Geometry check sheet. Reference: the model listing, model coordinates, mm. Face numbers are marked on the shaded views. A direction names the side the tool comes from. Round coordinates to 2 decimals unless told otherwise and drop trailing zeros. Order: outer loops, then holes, each group sorted by start corner. A loop starts at its lowest first (then second) coordinate and runs counter-clockwise, first axis right, second up. Notation, with made-up numbers: (5.5, -15) - (40.5, -15) arc R24 cw to (40.5, 24) - close; hole circle Ø11 at (36.5, 31). An arc over 180 degrees is marked (long way). Use a Markdown table: item, result. Add a question column.
(1) Mould release check, pull along Y, two halves, no side actions. Record for the marked faces 1, 2 and 3: released by +Y, released by -Y, zero draft, split by the parting line, or undercut.
(2) Access from +Z, -Z, +X, -X, +Y, -Y to the whole of each face (thin tool, end or side, straight path). Record for the marked faces 4, 5, 6 and 7.
(3) Gauge pin test, flat ends, axial feed: P1, Ø1, axis at x = 1.5, z = 19.5, coming from the -Y side; P2, Ø0.9, axis at x = 3, z = -4.5, coming from the +Y side; P3, Ø2.5, axis at x = 1.5, z = -2.5, coming from the +Y side. Record the tip position at first contact, or that the pin passes through.
(4) Section check D-D on z = 10. Record the boundary of the cut face in (x, y), then the cut area to 3 significant figures.
(5) Thickness scan on line 1 along Z through (x, y) = (4.35, -5.5); line 2 along Y through (x, z) = (3.55, 3.5); line 3 along Z through (x, y) = (3.9, -1). Record the ranges inside material, lowest first. Write a range as [from, to].
(6) Section check C-C on y = 6. Record the boundary of the cut face in (x, z), then the cut area to 3 significant figures.
(7) Section check A-A on x = 2.5. Record the boundary of the cut face in (y, z).
(8) Section check B-B on z = 33. Record the boundary of the cut face in (x, y), then the cut area to 3 significant figures.
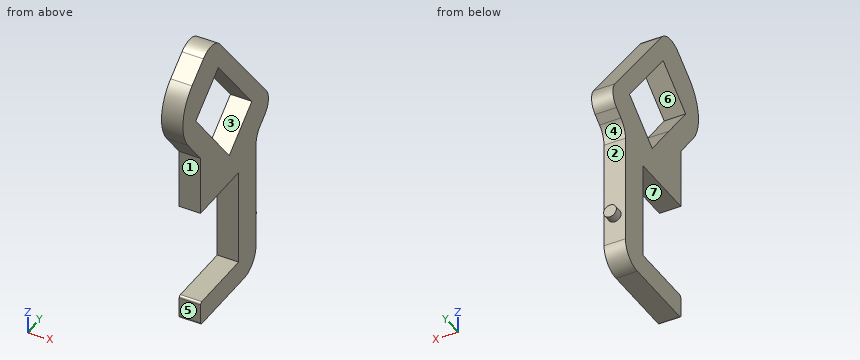
```python
from build123d import *

# Parameters (mm, degrees)
RESSALTO_EXTRUS_O2_DEPTH = 5
ESBO_O2_R                = 1.5
RESSALTO_EXTRUS_O3_DEPTH = 2


with BuildPart() as part:
    # Esboço1 → Ressalto-extrusão2 (new body)
    with BuildSketch(Plane(origin=(0, 0, 0), x_dir=(0, 0, -1), z_dir=(1, 0, 0))):
        with BuildLine():
            Line((11.9, -8), (16.485851709, -8))
            ThreePointArc((16.485851709, -8), (16.8394051, -7.853553391), (16.985851709, -7.5))
            Line((16.985851709, -7.5), (16.985851709, 10.3))
            ThreePointArc((16.985851709, 10.3), (15.521385615, 13.835533906), (11.985851709, 15.3))
            Line((11.985851709, 15.3), (-13.596583919, 15.3))
            ThreePointArc((-13.596583919, 15.3), (-15.768192588, 15.796210952), (-17.508770855, 17.186353684))
            Line((-17.508770855, 17.186353684), (-18.996698023, 19.055881768))
            ThreePointArc((-18.996698023, 19.055881768), (-21.674724782, 20.539376184), (-24.617364625, 19.694714264))
            Line((-24.617364625, 19.694714264), (-49.125535856, 0.18905712))
            ThreePointArc((-49.125535856, 0.18905712), (-50.977914533, -3.141239982), (-49.945591755, -6.809549569))
            Line((-49.945591755, -6.809549569), (-46.177076689, -11.612595572))
            ThreePointArc((-46.177076689, -11.612595572), (-39.507910608, -15.367707761), (-32.136832755, -13.307160494))
            Line((-32.136832755, -13.307160494), (-25.372753124, -8))
            Line((-25.372753124, -8), (-11.4, -8))
            Line((-11.4, -8), (-11.4, 8))
            Line((-11.4, 8), (11.4, 8))
            Line((11.4, 8), (11.4, -7.5))
            ThreePointArc((11.4, -7.5), (11.546446609, -7.853553391), (11.9, -8))
        make_face()
        Polygon((-27.25904201, -3), (-18.290200962, 4.037037037), (-25.882056579, 13.575936242), (-43.655854678, -0.569942233), (-36.227883057, -10.037037037), align=None, mode=Mode.SUBTRACT)
    extrude(amount=RESSALTO_EXTRUS_O2_DEPTH)

    # Esboço2 → Ressalto-extrusão3 (add)
    with BuildSketch(Plane(origin=(0, 15.3, 0), x_dir=(1, 0, 0), z_dir=(0, 1, 0))):
        with Locations(Location((2.5, 5.295851709, 0), (0, 0, 90))):
            Circle(ESBO_O2_R)
    extrude(amount=RESSALTO_EXTRUS_O3_DEPTH)


solid = part.part
```
Check sheet entries:
| question | item | result |
|---|---|---|
| 1 | face 1 | released by -Y |
| 1 | face 2 | released by +Y |
| 1 | face 3 | undercut |
| 2 | face 4 | +X, -X, +Y |
| 2 | face 5 | -Z, +X, -X, -Y |
| 2 | face 6 | +X, -X |
| 2 | face 7 | +X, -X, -Y |
| 3 | P1 | stops at y = -8 |
| 3 | P2 | stops at y = 17.3 |
| 3 | P3 | stops at y = 15.3 |
| 4 | outline | (0, 8) - (5, 8) - (5, 15.3) - (0, 15.3) - close |
| 4 | area | 36.5 mm2 |
| 5 | line 1 | z = [-16.99, -11.4], [11.4, 30.45], [39.79, 50.69] |
| 5 | line 2 | y = [8, 15.3] |
| 5 | line 3 | z = [-16.99, -11.4], [11.4, 24.71], [43.32, 50.21] |
| 6 | outline | (0, -16.99) - (5, -16.99) - (5, -11.4) - (0, -11.4) - close; (0, 11.4) - (5, 11.4) - (5, 19.85) - (0, 19.85) - close; (0, 35.4) - (5, 35.4) - (5, 41.82) - (0, 41.82) - close |
| 6 | area | 102 mm2 |
| 7 | outline | (-13.31, 32.14) - (-8, 25.37) - (-8, 11.4) - (8, 11.4) - (8, -11.4) - (-7.5, -11.4) arc R0.5 ccw to (-8, -11.9) - (-8, -16.49) arc R0.5 ccw to (-7.5, -16.99) - (10.3, -16.99) arc R5 ccw to (15.3, -11.99) - (15.3, -6.8) - (17.3, -6.8) - (17.3, -3.8) - (15.3, -3.8) - (15.3, 13.6) arc R5 cw to (17.19, 17.51) - (19.06, 19) arc R4 ccw to (19.69, 24.62) - (0.19, 49.13) arc R5 ccw to (-6.81, 49.95) - (-11.61, 46.18) arc R10 ccw to start; hole (-10.04, 36.23) - (4.04, 18.29) - (13.58, 25.88) - (-0.57, 43.66) - close |
| 8 | outline | (0, -13.91) - (5, -13.91) - (5, -7.5) - (0, -7.5) - close; (0, 7.91) - (5, 7.91) - (5, 13.02) - (0, 13.02) - close |
| 8 | area | 57.6 mm2 |
